Geometry check sheet. Reference: the model listing, model coordinates, mm. A direction names the side the tool comes from. Give positions to 0.01 mm unless a question says otherwise; leave off trailing zeros. Loops run counter-clockwise (first coordinate to the right, second up) from the corner with the lowest first, then second, coordinate; pieces in that order, holes last.
1. Release check for a two-part mould opening along Y. For faces 1 (the cylindrical face through (-21.874, 0.891, 2.916)), 2 (the flat face through (28, -35, 8)), 3 (the cylindrical face through (-9.63, 13.34, -0.03)) record: +Y half, -Y half, draft (parallel to the pull), parting line (faces both ways), or undercut.
2. Tool access check on faces 4 (the flat face through (-16, 25, 0)), 5 (the flat face through (0, -70, 1)), 6 (the flat face through (16, 25, 0)), 7 (the flat face through (0, 40, 0)), 8 (the flat face through (22, -33.8, 3.5)). Record the directions out of +Z, -Z, +X, -X, +Y, -Y that give a thin tool (end or side, any length) a straight path to the whole face; none if there is none.
3. Material ranges on L1, parallel to Y at x = -25.85, z = 13.5; L2, parallel to Y at x = 10, z = 0.45; L3, parallel to X at y = -18, z = 11.25, recorded low to high.
4. Go/stop test with flat-tipped pins: pin 1 Ø1.5 at (x, z) = (-22, 6) entering from +Y; pin 2 Ø5.5 at (y, z) = (20, 0) entering from +X; pin 3 Ø4 at (x, y) = (10, 15) entering from +Z; pin 4 Ø1.5 at (y, z) = (21.5, -0.5) entering from -X. Record where each tip stops, or that it passes through.
5. Cross-section at A-A, the plane y = 35. Record the cut outline in (x, z).
6. Cross-section at C-C, the plane x = 0. Record the cut outline in (y, z), plus the area to 3 significant figures.
7. Cross-section at B-B, the plane x = 10. Record the cut outline in (y, z), plus the area to 3 significant figures.
8. Cross-section at D-D, the plane y = -36. Record the cut outline in (x, z), plus the area to 3 significant figures.
from build123d import *

# Parameters (mm, degrees)
SKETCH1_W            = 32
SKETCH1_H            = 5
BOSS_EXTRUDE1_DEPTH  = 40
M3_CLEARANCE_HOLE3_D = 3.4
SKETCH4_W            = 46
SKETCH4_H            = 5
BOSS_EXTRUDE2_DEPTH  = 70
SKETCH5_W            = 5
SKETCH5_H            = 20
BOSS_EXTRUDE3_DEPTH  = 70
M3_CLEARANCE_HOLE1_D = 3.4
M3_CLEARANCE_HOLE2_D = 3.4
FILLET2_R            = 10
FILLET4_SIZE         = 2


with BuildPart() as part:
    # Sketch1 → Boss-Extrude1 (new body)
    with BuildSketch(Plane(origin=(0, 0, 0), x_dir=(1, 0, 0), z_dir=(0, 1, 0))):
        Rectangle(SKETCH1_W, SKETCH1_H)
    extrude(amount=BOSS_EXTRUDE1_DEPTH)

    # M3 Clearance Hole3 (through all)
    with Locations(Plane.XY.offset(2.5)):
        with Locations((-10, 35), (10, 35), (10, 15), (-10, 15)):
            Hole(M3_CLEARANCE_HOLE3_D / 2)

    # Sketch4 → Boss-Extrude2 (add)
    with BuildSketch(Plane(origin=(0, 0, 0), x_dir=(1, 0, 0), z_dir=(0, 1, 0))):
        Rectangle(SKETCH4_W, SKETCH4_H)
    extrude(amount=-BOSS_EXTRUDE2_DEPTH)

    # Sketch5 → Boss-Extrude3 (add)
    with BuildSketch(Plane(origin=(0, 0, 0), x_dir=(1, 0, 0), z_dir=(0, 1, 0))):
        with Locations((25.5, -7.5)):
            Rectangle(SKETCH5_W, SKETCH5_H)
        with Locations((-25.5, -7.5)):
            Rectangle(SKETCH5_W, SKETCH5_H)
    extrude(amount=-BOSS_EXTRUDE3_DEPTH)

    # M3 Clearance Hole1 (through all)
    with Locations(Plane(origin=(28, 0, 0), x_dir=(0, 0, -1), z_dir=(1, 0, 0))):
        with Locations((-13.5, -5), (-13.5, -65)):
            Hole(M3_CLEARANCE_HOLE1_D / 2)

    # M3 Clearance Hole2 (through all)
    with Locations(Plane(origin=(0, 0, -2.5), x_dir=(-1, 0, 0), z_dir=(0, 0, -1))):
        with Locations((-10, -23), (10, -23), (0, -33), (-10, -63), (10, -63)):
            Hole(M3_CLEARANCE_HOLE2_D / 2)

    # Fillet2
    fillet2_edges = [part.edges().sort_by_distance(p)[0] for p in [
        (-16, 0, 0),
        (16, 0, 0),
    ]]
    fillet(fillet2_edges, radius=FILLET2_R)

    # Fillet4
    fillet4_edges = [part.edges().sort_by_distance(p)[0] for p in [
        (-23, -34.769696007, 2.5),
        (23, -34.769696007, 2.5),
    ]]
    chamfer(fillet4_edges, length=FILLET4_SIZE)


solid = part.part
Result:
1. face 1: +Y half
1. face 2: draft
1. face 3: undercut
2. face 4: +Z, -Z, -X, +Y
2. face 5: +Z, -Z, +X, -X, -Y
2. face 6: +Z, -Z, +X, +Y
2. face 7: +Z, -Z, +X, -X, +Y
2. face 8: +Z, +Y, -Y
3. L1: y = -70 to -66.7, -63.3 to -6.7, -3.3 to 0
3. L2: y = -70 to -64.7, -61.3 to -24.7, -21.3 to 13.3, 16.7 to 33.3, 36.7 to 40
3. L3: x = -28 to -23, 23 to 28
4. pin 1: passes through
4. pin 2: stops at x = 16
4. pin 3: stops at z = 2.5
4. pin 4: stops at x = -16
5. outline: (-16, -2.5) - (-11.7, -2.5) - (-11.7, 2.5) - (-16, 2.5) - close; (-8.3, -2.5) - (8.3, -2.5) - (8.3, 2.5) - (-8.3, 2.5) - close; (11.7, -2.5) - (16, -2.5) - (16, 2.5) - (11.7, 2.5) - close
6. outline: (-70, -2.5) - (-34.7, -2.5) - (-34.7, 2.5) - (-70, 2.5) - close; (-31.3, -2.5) - (40, -2.5) - (40, 2.5) - (-31.3, 2.5) - close
6. area: 533 mm2
7. outline: (-70, -2.5) - (-64.7, -2.5) - (-64.7, 2.5) - (-70, 2.5) - close; (-61.3, -2.5) - (-24.7, -2.5) - (-24.7, 2.5) - (-61.3, 2.5) - close; (-21.3, -2.5) - (13.3, -2.5) - (13.3, 2.5) - (-21.3, 2.5) - close; (16.7, -2.5) - (33.3, -2.5) - (33.3, 2.5) - (16.7, 2.5) - close; (36.7, -2.5) - (40, -2.5) - (40, 2.5) - (36.7, 2.5) - close
7. area: 482 mm2
8. outline: (-28, -2.5) - (28, -2.5) - (28, 17.5) - (23, 17.5) - (23, 4.5) - (21, 2.5) - (-21, 2.5) - (-23, 4.5) - (-23, 17.5) - (-28, 17.5) - close
8. area: 434 mm2
